```python
from build123d import *

# Parameters (mm, degrees)
SKETCH3_R           = 1.3
BOSS_EXTRUDE2_DEPTH = 5
SKETCH5_R           = 35
BOSS_EXTRUDE4_DEPTH = 28.1
CHAMFER2_SIZE       = 2
SKETCH6_R           = 25
BOSS_EXTRUDE5_DEPTH = 3
CHAMFER3_SIZE       = 1
SKETCH7_R           = 16
BOSS_EXTRUDE6_DEPTH = 20
SKETCH8_R           = 3.55
BOSS_EXTRUDE7_DEPTH = 2
FILLET1_R           = 2
SKETCH9_R           = 1.3
BOSS_EXTRUDE8_DEPTH = 8
SKETCH11_R          = 1.3
BOSS_EXTRUDE9_DEPTH = 1.9


with BuildPart() as part:
    # Sketch3 → Boss-Extrude2 (new body)
    with BuildSketch(Plane(origin=(0, 0, 0), x_dir=(1, 0, 0), z_dir=(0, 1, 0))):
        with BuildLine():
            ThreePointArc((-46.25, 30), (-47.664213562, 29.414213562), (-48.25, 28))
            ThreePointArc((-48.25, 28), (-49.607700542, 0), (-48.25, -28))
            ThreePointArc((-48.25, -28), (-47.664213562, -29.414213562), (-46.25, -30))
            ThreePointArc((-46.25, -30), (-0.19378614, -33.636910917), (41.856895399, -14.502069967))
            ThreePointArc((41.856895399, -14.502069967), (49.25, 0), (41.856895399, 14.502069967))
            ThreePointArc((41.856895399, 14.502069967), (-0.19378614, 33.636910917), (-46.25, 30))
        make_face()
        with Locations((-46.25, 28)):
            Circle(SKETCH3_R, mode=Mode.SUBTRACT)
        with Locations((-46.25, -28)):
            Circle(SKETCH3_R, mode=Mode.SUBTRACT)
        with Locations((23.75, 20)):
            Circle(SKETCH3_R, mode=Mode.SUBTRACT)
        with Locations((23.75, -20)):
            Circle(SKETCH3_R, mode=Mode.SUBTRACT)
    extrude(amount=BOSS_EXTRUDE2_DEPTH)

    # Sketch5 → Boss-Extrude4 (add)
    with BuildSketch(Plane(origin=(0, 5, 0), x_dir=(1, 0, 0), z_dir=(0, 1, 0))):
        with Locations((-14.607700542, 0)):
            Circle(SKETCH5_R)
    extrude(amount=BOSS_EXTRUDE4_DEPTH)

    # Chamfer2
    chamfer2_edges = [part.edges().sort_by_distance(p)[0] for p in [
        (-49.607700542, 33.1, 0),
    ]]
    chamfer(chamfer2_edges, length=CHAMFER2_SIZE)

    # Sketch6 → Boss-Extrude5 (add)
    with BuildSketch(Plane.XZ):
        with Locations((-14.607700542, 0)):
            Circle(SKETCH6_R)
    extrude(amount=BOSS_EXTRUDE5_DEPTH)

    # Chamfer3
    chamfer3_edges = [part.edges().sort_by_distance(p)[0] for p in [
        (-39.607700542, -3, 0),
    ]]
    chamfer(chamfer3_edges, length=CHAMFER3_SIZE)

    # Sketch7 → Boss-Extrude6 (add)
    with BuildSketch(Plane.XZ):
        with Locations((30.892299458, 0)):
            Circle(SKETCH7_R)
    extrude(amount=BOSS_EXTRUDE6_DEPTH)

    # Sketch8 → Boss-Extrude7 (add)
    with BuildSketch(Plane.XZ.offset(20)):
        with Locations((30.892299458, 0)):
            Circle(SKETCH8_R)
    extrude(amount=BOSS_EXTRUDE7_DEPTH)

    # Fillet1
    fillet1_edges = [part.edges().sort_by_distance(p)[0] for p in [
        (14.892299458, -20, 0),
    ]]
    fillet(fillet1_edges, radius=FILLET1_R)

    # Sketch9 → Boss-Extrude8 (add)
    with BuildSketch(Plane.XZ):
        Polygon((22.667730051, -18.647708701), (22.037746407, -20.261127619), (23.120016356, -21.613418919), (24.832269949, -21.352291299), (25.462253593, -19.738872381), (24.379983644, -18.386581081), align=None)
        with Locations((23.75, -20)):
            Circle(SKETCH9_R, mode=Mode.SUBTRACT)
        Polygon((-47.27859803, -26.606448389), (-47.971150112, -28.194016218), (-46.942552082, -29.58756783), (-45.22140197, -29.393551611), (-44.528849888, -27.805983782), (-45.557447918, -26.41243217), align=None)
        with Locations((-46.25, -28)):
            Circle(SKETCH9_R, mode=Mode.SUBTRACT)
        Polygon((-47.117302489, 29.499261949), (-47.98205018, 27.998524986), (-47.11474769, 26.499263037), (-45.382697511, 26.500738051), (-44.51794982, 28.001475014), (-45.38525231, 29.500736963), align=None)
        with Locations((-46.25, 28)):
            Circle(SKETCH9_R, mode=Mode.SUBTRACT)
        Polygon((22.220041565, 20.811928069), (22.281870449, 19.080981163), (23.811828884, 18.269053095), (25.279958435, 19.188071931), (25.218129551, 20.919018837), (23.688171116, 21.730946905), align=None)
        with Locations((23.75, 20)):
            Circle(SKETCH9_R, mode=Mode.SUBTRACT)
    extrude(amount=BOSS_EXTRUDE8_DEPTH)

    # Sketch11 → Boss-Extrude9 (add)
    with BuildSketch(Plane(origin=(0, -8, 0), x_dir=(-1, 0, 0), z_dir=(0, -1, 0))):
        with BuildLine():
            ThreePointArc((46.25, 30), (9.738587829, 34.807277641), (-25.746736736, 24.959187593))
            ThreePointArc((-25.746736736, 24.959187593), (-27.89999608, 19.965760464), (-24.474790494, 15.742159277))
            ThreePointArc((-24.474790494, 15.742159277), (-13.920811193, 0.984167698), (-22.698167109, -14.894837865))
            ThreePointArc((-22.698167109, -14.894837865), (-27.065884089, -19.065715062), (-25.746736736, -24.959187593))
            ThreePointArc((-25.746736736, -24.959187593), (9.738587829, -34.807277641), (46.25, -30))
            ThreePointArc((46.25, -30), (47.664213562, -29.414213562), (48.25, -28))
            ThreePointArc((48.25, -28), (49.607700542, 0), (48.25, 28))
            ThreePointArc((48.25, 28), (47.664213562, 29.414213562), (46.25, 30))
        make_face()
        with Locations((-23.75, 20)):
            Circle(SKETCH11_R, mode=Mode.SUBTRACT)
        with Locations((-23.75, -20)):
            Circle(SKETCH11_R, mode=Mode.SUBTRACT)
        with Locations((46.25, -28)):
            Circle(SKETCH11_R, mode=Mode.SUBTRACT)
        with Locations((46.25, 28)):
            Circle(SKETCH11_R, mode=Mode.SUBTRACT)
    extrude(amount=BOSS_EXTRUDE9_DEPTH)


solid = part.part
```
Input: part model. Units: mm. Frame: model coordinates. A direction names the side the tool comes from. Coordinates: 2 decimals unless noted, no trailing zeros. Write each loop counter-clockwise with the first axis right and the second up, starting at its lowest first coordinate (ties: lowest second). Pieces come first, ordered by that corner, then holes.
1) Mould query, pull axis Z, two halves, no side actions, for faces 1 (the cylindrical face through (13.94, -8.94, -1.25)), 2 (the flat face through (22, 5, 0)), 3 (the cylindrical face through (-0.84, 2.46, 33.75)), 4 (the cylindrical face through (27.04, -8.94, 18.98)). Classes: pulls with the +Z half, pulls with the -Z half, needs draft (parallel to the pull), parting line crosses it, or undercut.
2) Material intervals for line 1 along Z through (x, y) = (-46.25, 2); line 2 along Y through (x, z) = (-44.5, -2.5); line 3 along Z through (x, y) = (-46.25, -4.75), sorted ascending.
3) Pin query (flat end, axial travel): pin 1 Ø4 at (x, z) = (5.5, -0.5) entering from -Y; pin 2 Ø10 at (x, y) = (-11, 17) entering from +Z; pin 3 Ø2 at (x, z) = (23.75, -20) entering from +Y; pin 4 Ø3 at (x, z) = (23.75, -20) entering from +Y. Return the tip coordinate at first contact, or that it passes through.
4) Section A-A on y = 9.5. Output: boundary loops of the cut face in (x, z).
5) Set-up query: faces 5 (the cylindrical face through (-42.38, 17.87, 21.3)), 6 (the cylindrical face through (-33.03, -0.99, 16.9)), 7 (the cylindrical face through (-47.68, 2.46, 29.4)), 8 (the cylindrical face through (18.2, -8.87, -9.74)). Return all of +Z, -Z, +X, -X, +Y, -Y with unobstructed straight access to the full face (end or side cutting, diameter ignored); none if empty.
Check result:
1. face 1: undercut
1. face 2: needs draft
1. face 3: pulls with the +Z half
1. face 4: undercut
2. line 1: z = -30 to -29.3, -26.7 to 26.7, 29.3 to 30
2. line 2: y = -9.9 to -8, 0 to 33.1
2. line 3: z = -29.51 to -29.3, -26.7 to -26.49, 26.5 to 26.7, 29.3 to 29.5
3. pin 1: stops at y = -9.9
3. pin 2: stops at z = 35
3. pin 3: passes through
3. pin 4: stops at y = 5
4. outline: circle Ø70 at (-14.61, 0)
5. face 5: +Y
5. face 6: none
5. face 7: +Z, -X, +Y, -Y
5. face 8: -Y
